The model under review builds one solid part; all positions refer to its coordinate system, in mm. Coordinates: 2 decimals unless noted, no trailing zeros. Order: outer loops, then holes, each group sorted by start corner. A loop starts at its lowest first (then second) coordinate and runs counter-clockwise, first axis right, second up. Notation, with made-up numbers: M 69.25,-5.75 L 102.25,-5.75 A23 ccw 102.25,7.25 Z; hole C 20,79.5 d1. An arc over 180 degrees is marked long. One line per item, written item: value.
```python
from build123d import *

# Parameters (mm, degrees)
SKETCH_3_W                  = 60
SKETCH_3_H                  = 30
EXTRUDE_2_DEPTH             = 3
HOLE_WIZARD_M84_D           = 6.8
HOLE_WIZARD_M84_CSINK_D     = 8.05
HOLE_WIZARD_M84_CSINK_ANGLE = 90


with BuildPart() as part:
    # Эскиз3 → Бобышка-Вытянуть2 (new, symmetric)
    with BuildSketch(Plane(origin=(56, 0, 0), x_dir=(0, 0, -1), z_dir=(1, 0, 0))):
        with Locations((0, 70)):
            Rectangle(SKETCH_3_W, SKETCH_3_H)
    extrude(amount=EXTRUDE_2_DEPTH, both=True)

    # Отверстие обработанное метчиком M84 (through all)
    with Locations(Plane(origin=(59, 0, 0), x_dir=(0, 0, -1), z_dir=(1, 0, 0))):
        with Locations((-15, 70), (15, 70)):
            CounterSinkHole(HOLE_WIZARD_M84_D / 2, HOLE_WIZARD_M84_CSINK_D / 2, counter_sink_angle=HOLE_WIZARD_M84_CSINK_ANGLE)


solid = part.part
```
(1) Mouldability with a two-part tool opening along Y and no side actions: class faces 1 (the cylindrical face through (55.65, 66.68, 14.26)), 2 (the cylindrical face through (55.65, 66.68, -15.74)), 3 (the flat face through (56, 85, 0)), 4 (the flat face through (56, 70, 30)) as +Y half, -Y half, draft (parallel to the pull), parting line (faces both ways), or undercut.
Geometry results:
face 1: undercut
face 2: undercut
face 3: +Y half
face 4: draft
(2) We need section A-A, the plane z = 15. State the section outline as (x, y) points (3 decimals).
Geometry results:
outline: M 53,55 L 59,55 L 59,65.975 L 58.375,66.6 L 53,66.6 Z; M 53,73.4 L 58.375,73.4 L 59,74.025 L 59,85 L 53,85 Z
(3) Insertion check: pin 1 Ø8 at (y, z) = (70, 15) entering from +X (3 decimals). The pin has a flat end and moves straight along its axis. Give the tip position at first contact, or say it passes through.
Geometry results:
pin 1: stops at x = 58.975
(4) For L1, parallel to Z at x = 56.05, y = 70; L2, parallel to Y at x = 57.2, z = -15; L3, parallel to Z at x = 57.85, y = 71.25, list the stretches that pass through material, from the lowest coordinate up.
Geometry results:
L1: z = -30 to -18.4, -11.6 to 11.6, 18.4 to 30
L2: y = 55 to 66.6, 73.4 to 85
L3: z = -30 to -18.16, -11.84 to 11.84, 18.16 to 30
(5) We need section C-C, the plane x = 54.25. State the section outline as (y, z) points.
Geometry results:
outline: M 55,-30 L 85,-30 L 85,30 L 55,30 Z; hole C 70,-15 d6.8; hole C 70,15 d6.8
(6) We need section B-B, the plane y = 70. State the section outline as (x, z) points (3 decimals), plus the area to 3 significant figures.
Geometry results:
outline: M 53,-30 L 59,-30 L 59,-19.025 L 58.375,-18.4 L 53,-18.4 Z; M 53,-11.6 L 58.375,-11.6 L 59,-10.975 L 59,10.975 L 58.375,11.6 L 53,11.6 Z; M 53,18.4 L 58.375,18.4 L 59,19.025 L 59,30 L 53,30 Z
area: 278 mm2
